from build123d import *

# Parameters (mm, degrees)
BOSS_EXTRUDE1_DEPTH = 50
SKETCH2_W           = 7
SKETCH2_H           = 8
BOSS_EXTRUDE2_DEPTH = 50
SKETCH2_3_W         = 7
SKETCH2_3_H         = 8
BOSS_EXTRUDE3_DEPTH = 18
SKETCH3_W           = 10
SKETCH3_H           = 63
SKETCH3_W_2         = 7
SKETCH3_H_2         = 8
BOSS_EXTRUDE4_DEPTH = 82
FILLET1_R           = 5
SKETCH4_W           = 49
SKETCH4_H           = 25.5
CUT_EXTRUDE1_DEPTH  = 63
SKETCH5_W           = 25.5
SKETCH5_H           = 10
SKETCH5_H_2         = 12
BOSS_EXTRUDE5_DEPTH = 49
CUT_EXTRUDE2_DEPTH  = 25.5
SKETCH6_R           = 1.75
CUT_EXTRUDE3_DEPTH  = 5
SKETCH6_6_R         = 0.75
CUT_EXTRUDE4_DEPTH  = 15
SKETCH8_W           = 18
SKETCH8_H           = 9.5
CUT_EXTRUDE5_DEPTH  = 40
SKETCH9_W           = 40
SKETCH9_H           = 25.5
CUT_EXTRUDE6_DEPTH  = 110.982953225
SKETCH10_W          = 32
SKETCH10_H          = 88.5
CUT_EXTRUDE7_DEPTH  = 111.174861016
SKETCH11_W          = 50
SKETCH11_H          = 63
CUT_EXTRUDE8_DEPTH  = 105.797423632
SKETCH12_W          = 25.5
SKETCH12_H          = 35
BOSS_EXTRUDE7_DEPTH = 10
SKETCH12_3_R        = 10
CUT_EXTRUDE9_DEPTH  = 107.716915248
SKETCH13_W          = 42.5
SKETCH13_H          = 88.5
CUT_EXTRUDE10_DEPTH = 25
SKETCH14_W          = 25
SKETCH14_H          = 28
CUT_EXTRUDE11_DEPTH = 96.433222727
SKETCH15_W          = 25
SKETCH15_H          = 60.5
CUT_EXTRUDE12_DEPTH = 71.25311381
SKETCH16_W          = 10
SKETCH16_H          = 35
CUT_EXTRUDE13_DEPTH = 68.633201906
SKETCH17_W          = 15
SKETCH17_H          = 35
BOSS_EXTRUDE8_DEPTH = 3
BOSS_EXTRUDE9_DEPTH = 10
SKETCH19_R          = 1.25
CUT_EXTRUDE14_DEPTH = 54.574714185
FILLET4_R           = 5


with BuildPart() as part:
    # Sketch1 → Boss-Extrude1 (new body)
    with BuildSketch(Plane.XY):
        with BuildLine():
            Line((-2.25, -8), (-4.25, -8))
            ThreePointArc((-4.25, -8), (-3.25, -8.5), (-2.25, -8))
        make_face()
        Polygon((10, -25.5), (10, 0), (0, 0), (-18, 0), (-18, -8), (0, -8), (0, -17.5), (-18, -17.5), (-18, -25.5), align=None)
    extrude(amount=BOSS_EXTRUDE1_DEPTH)

    # Sketch2 → Boss-Extrude2 (add)
    with BuildSketch(Plane(origin=(0, 0, 0), x_dir=(0, 0, -1), z_dir=(1, 0, 0))):
        Polygon((7, 0), (0, 0), (0, -8), (2.25, -8), (4.25, -8), (7, -8), align=None)
        Polygon((0, -8), (0, 0), (-10, 0), (-10, -25.5), (0, -25.5), (0, -17.5), align=None)
        with Locations((3.5, -21.5)):
            Rectangle(SKETCH2_W, SKETCH2_H)
        with BuildLine():
            Line((4.25, -8), (2.25, -8))
            ThreePointArc((2.25, -8), (3.25, -8.5), (4.25, -8))
        make_face()
    extrude(amount=BOSS_EXTRUDE2_DEPTH)

    # Sketch2<3> → Boss-Extrude3 (add)
    with BuildSketch(Plane(origin=(0, 0, 0), x_dir=(0, 0, -1), z_dir=(1, 0, 0))):
        Polygon((7, 0), (0, 0), (0, -8), (2.25, -8), (4.25, -8), (7, -8), align=None)
        with Locations((3.5, -21.5)):
            Rectangle(SKETCH2_3_W, SKETCH2_3_H)
    extrude(amount=-BOSS_EXTRUDE3_DEPTH)

    # Sketch3 → Boss-Extrude4 (add)
    with BuildSketch(Plane(origin=(50, 0, 0), x_dir=(0, 0, -1), z_dir=(1, 0, 0))):
        Polygon((32.5, -17.5), (7, -17.5), (7, -25.5), (0, -25.5), (0, -88.5), (32.5, -88.5), align=None)
        with Locations((-5, -57)):
            Rectangle(SKETCH3_W, SKETCH3_H)
        with Locations((3.5, -21.5)):
            Rectangle(SKETCH3_W_2, SKETCH3_H_2)
        with Locations((-5, -21.5)):
            Rectangle(SKETCH3_W, SKETCH3_H_2)
    extrude(amount=-BOSS_EXTRUDE4_DEPTH)

    # Fillet1
    fillet1_edges = [part.edges().sort_by_distance(p)[0] for p in [
        (-32, -17.5, -11.25),
        (-32, -53, -32.5),
        (9, -17.5, -32.5),
    ]]
    fillet(fillet1_edges, radius=FILLET1_R)

    # Sketch4 → Cut-Extrude1 (cut)
    with BuildSketch(Plane.XZ.offset(88.5)):
        with Locations((25.5, -2.75)):
            Rectangle(SKETCH4_W, SKETCH4_H)
    extrude(amount=-CUT_EXTRUDE1_DEPTH, mode=Mode.SUBTRACT)

    # Sketch5 → Boss-Extrude5 (add)
    with BuildSketch(Plane(origin=(50, 0, 0), x_dir=(0, 0, -1), z_dir=(1, 0, 0))):
        with Locations((2.75, -30.5)):
            Rectangle(SKETCH5_W, SKETCH5_H)
        with Locations((2.75, -82.5)):
            Rectangle(SKETCH5_W, SKETCH5_H_2)
    extrude(amount=-BOSS_EXTRUDE5_DEPTH)

    # Sketch7 → Cut-Extrude2 (cut)
    with BuildSketch(Plane.XY.offset(10)):
        Polygon((1, -35.5), (27, -35.5), (27, -25.5), (50, -25.5), (50, -88.5), (27, -88.5), (27, -76.5), (1, -76.5), align=None)
    extrude(amount=-CUT_EXTRUDE2_DEPTH, mode=Mode.SUBTRACT)

    # Sketch6 → Cut-Extrude3 (cut)
    with BuildSketch(Plane(origin=(27, 0, 0), x_dir=(0, 0, -1), z_dir=(1, 0, 0))):
        with Locations((0.25, -81.5)):
            Circle(SKETCH6_R)
        with Locations((10.25, -81.5)):
            Circle(SKETCH6_R)
        with Locations((10.25, -32.5)):
            Circle(SKETCH6_R)
        with Locations((0.25, -32.5)):
            Circle(SKETCH6_R)
    extrude(amount=-CUT_EXTRUDE3_DEPTH, mode=Mode.SUBTRACT)

    # Sketch6<6> → Cut-Extrude4 (cut)
    with BuildSketch(Plane(origin=(27, 0, 0), x_dir=(0, 0, -1), z_dir=(1, 0, 0))):
        with Locations((0.25, -81.5)):
            Circle(SKETCH6_6_R)
        with Locations((10.25, -81.5)):
            Circle(SKETCH6_6_R)
        with Locations((10.25, -32.5)):
            Circle(SKETCH6_6_R)
        with Locations((0.25, -32.5)):
            Circle(SKETCH6_6_R)
    extrude(amount=-CUT_EXTRUDE4_DEPTH, mode=Mode.SUBTRACT)

    # Sketch8 → Cut-Extrude5 (cut)
    with BuildSketch(Plane(origin=(0, 0, -7), x_dir=(-1, 0, 0), z_dir=(0, 0, -1))):
        with Locations((9, -12.75)):
            Rectangle(SKETCH8_W, SKETCH8_H)
    extrude(amount=-CUT_EXTRUDE5_DEPTH, mode=Mode.SUBTRACT)

    # Sketch9 → Cut-Extrude6 (cut, through all)
    with BuildSketch(Plane(origin=(10, 0, 0), x_dir=(0, 0, -1), z_dir=(1, 0, 0))):
        with Locations((-30, -12.75)):
            Rectangle(SKETCH9_W, SKETCH9_H)
    extrude(amount=-CUT_EXTRUDE6_DEPTH, mode=Mode.SUBTRACT)

    # Sketch10 → Cut-Extrude7 (cut, through all)
    with BuildSketch(Plane.XY.offset(10)):
        with Locations((-16, -44.25)):
            Rectangle(SKETCH10_W, SKETCH10_H)
    extrude(amount=-CUT_EXTRUDE7_DEPTH, mode=Mode.SUBTRACT)

    # Sketch11 → Cut-Extrude8 (cut, through all)
    with BuildSketch(Plane.XY.offset(-15.5)):
        with Locations((25, -57)):
            Rectangle(SKETCH11_W, SKETCH11_H)
    extrude(amount=CUT_EXTRUDE8_DEPTH, mode=Mode.SUBTRACT)

    # Sketch12 → Boss-Extrude7 (add)
    with BuildSketch(Plane.ZY):
        with Locations((-2.75, -43)):
            Rectangle(SKETCH12_W, SKETCH12_H)
    extrude(amount=-BOSS_EXTRUDE7_DEPTH)

    # Sketch12<3> → Cut-Extrude9 (cut, through all)
    with BuildSketch(Plane.ZY):
        with Locations(Location((-5.5, -42.5, 0), (0, 0, 270))):
            Circle(SKETCH12_3_R)
    extrude(amount=-CUT_EXTRUDE9_DEPTH, mode=Mode.SUBTRACT)

    # Sketch13 → Cut-Extrude10 (cut)
    with BuildSketch(Plane(origin=(50, 0, 0), x_dir=(0, 0, -1), z_dir=(1, 0, 0))):
        with Locations((11.25, -44.25)):
            Rectangle(SKETCH13_W, SKETCH13_H)
    extrude(amount=-CUT_EXTRUDE10_DEPTH, mode=Mode.SUBTRACT)

    # Sketch14 → Cut-Extrude11 (cut, through all)
    with BuildSketch(Plane.XY.offset(-15.5)):
        with Locations((12.5, -74.5)):
            Rectangle(SKETCH14_W, SKETCH14_H)
    extrude(amount=-CUT_EXTRUDE11_DEPTH, mode=Mode.SUBTRACT)

    # Sketch15 → Cut-Extrude12 (cut, through all)
    with BuildSketch(Plane(origin=(0, 0, -7), x_dir=(-1, 0, 0), z_dir=(0, 0, -1))):
        with Locations((-12.5, -30.25)):
            Rectangle(SKETCH15_W, SKETCH15_H)
    extrude(amount=CUT_EXTRUDE12_DEPTH, mode=Mode.SUBTRACT)

    # Sketch16 → Cut-Extrude13 (cut, through all)
    with BuildSketch(Plane(origin=(0, 0, -7), x_dir=(-1, 0, 0), z_dir=(0, 0, -1))):
        with Locations((-5, -43)):
            Rectangle(SKETCH16_W, SKETCH16_H)
    extrude(amount=-CUT_EXTRUDE13_DEPTH, mode=Mode.SUBTRACT)

    # Sketch17 → Boss-Extrude8 (add)
    with BuildSketch(Plane(origin=(0, -17.5, 0), x_dir=(1, 0, 0), z_dir=(0, 1, 0))):
        with Locations((17.5, -17.5)):
            Rectangle(SKETCH17_W, SKETCH17_H)
    extrude(amount=-BOSS_EXTRUDE8_DEPTH)

    # Sketch18 → Boss-Extrude9 (add)
    with BuildSketch(Plane(origin=(25, 0, 0), x_dir=(0, 0, -1), z_dir=(1, 0, 0))):
        Polygon((-10, -17.5), (-35, -17.5), (-35, -20.5), (-10, -20.5), (0, -20.5), (0, -17.5), align=None)
    extrude(amount=BOSS_EXTRUDE9_DEPTH)

    # Sketch19 → Cut-Extrude14 (cut, through all)
    with BuildSketch(Plane.XZ.offset(20.5)):
        Polygon((35, 0), (35, 22), (25, 22), (25, 10), (25, 0), align=None)
        with Locations(Location((32, 25, 0), (0, 0, 270))):
            Circle(SKETCH19_R)
        with Locations(Location((32, 31.5, 0), (0, 0, 270))):
            Circle(SKETCH19_R)
    extrude(amount=-CUT_EXTRUDE14_DEPTH, mode=Mode.SUBTRACT)

    # Fillet4
    fillet4_edges = [part.edges().sort_by_distance(p)[0] for p in [
        (10, -19, 10),
        (17.5, -20.5, 10),
        (10, -19, 35),
        (17.5, -17.5, 10),
        (25, -19, 22),
    ]]
    fillet(fillet4_edges, radius=FILLET4_R - 0.0001)  # a hair under: the kernel refuses the full size


solid = part.part
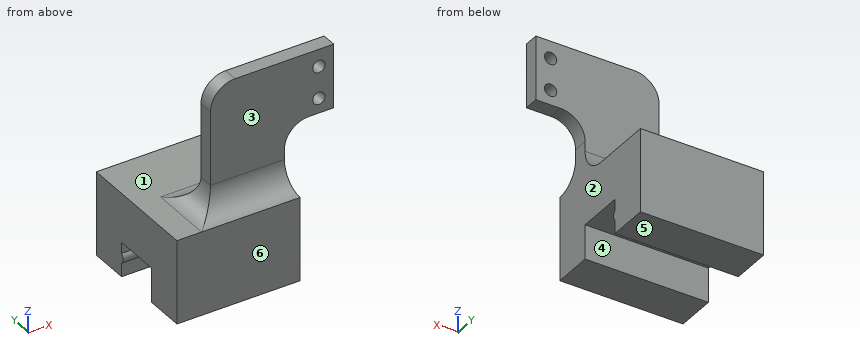
Check sheet for the modelled part. Datum: model origin and axes. Units: mm. Face numbers are marked on the shaded views. A direction names the side the tool comes from. Round coordinates to 2 decimals unless told otherwise and drop trailing zeros. Loops run counter-clockwise (first coordinate to the right, second up) from the corner with the lowest first, then second, coordinate; pieces in that order, holes last. Notation, with made-up numbers: (61.5, 85.25) -> (94.5, 85.25) arc R26 cw to (94.5, 118.25) -> close; hole circle Ø8 at (14.5, 89.5). An arc over 180 degrees is marked (long way). Put each result on its own line as item: value. Start each with the question number.
1. Section check C-C (y = -20). Enter the section's corners in (x, z), plus the area to 3 significant figures.
2. Scan lines: probe 1 along X at (y, z) = (-19.2, 25); probe 2 along Y at (x, z) = (21.5, 31); probe 3 along X at (y, z) = (-22, -2). Record each from-to range of solid material in increasing order.
3. Gauge pin test, flat ends, axial feed: pin 1 (1.5 mm diameter, centred on x = 22.5, z = 12.5, fed in from -Y); pin 2 (10 mm diameter, centred on x = 19.5, z = 24.5, fed in from -Y); pin 3 (0.9 mm diameter, centred on y = -18.5, z = 21.5, fed in from -X). Record the tip position at first contact, or that the pin passes through.
4. Section check A-A (z = 25). Enter the section's corners in (x, y), plus the area to 3 significant figures.
5. Section check B-B (x = 32). Enter the section's corners in (y, z).
6. Draft check along Y on the marked faces 4, 5 and 6. Enter one of: +Y half, -Y half, draft (parallel to the pull), parting line (faces both ways), or undercut.
7. Access from +Z, -Z, +X, -X, +Y, -Y to the whole of each face (thin tool, end or side, straight path). Record for the marked faces 1, 2 and 3.
Findings:
1. outline: (0, -7) -> (25, -7) -> (25, 17) arc R5 cw to (30, 22) -> (35, 22) -> (35, 35) -> (15, 35) arc R5 ccw to (10, 30) -> (10, 15) arc R5 cw to (5, 10) -> (0, 10) -> close; hole circle Ø2.5 at (32, 25); hole circle Ø2.5 at (32, 31.5)
1. area: 926 mm^2
2. probe 1: x = 10 to 30.75, 33.25 to 35
2. probe 2: y = -20.5 to -17.5
2. probe 3: x = 0 to 25
3. pin 1: stops at y = -21.7
3. pin 2: stops at y = -20.5
3. pin 3: stops at x = 10
4. outline: (10, -20.5) -> (30.75, -20.5) -> (30.75, -17.5) -> (10, -17.5) -> close; (33.25, -20.5) -> (35, -20.5) -> (35, -17.5) -> (33.25, -17.5) -> close
4. area: 67.5 mm^2
5. outline: (-20.5, 22) -> (-17.5, 22) -> (-17.5, 23.75) -> (-20.5, 23.75) -> close; (-20.5, 26.25) -> (-17.5, 26.25) -> (-17.5, 30.25) -> (-20.5, 30.25) -> close; (-20.5, 32.75) -> (-17.5, 32.75) -> (-17.5, 35) -> (-20.5, 35) -> close
6. face 4: undercut
6. face 5: draft
6. face 6: -Y half
7. face 1: +Z, -X, +Y
7. face 2: -Z, +X, +Y, -Y
7. face 3: +Z, +X, -X, -Y
